Part print with two shaded views. Sizes in mm from the minimum x, y, z corner. Round coordinates to 2 decimals unless told otherwise and drop trailing zeros. Loops run counter-clockwise (first coordinate to the right, second up) from the corner with the lowest first, then second, coordinate; pieces in that order, holes last.
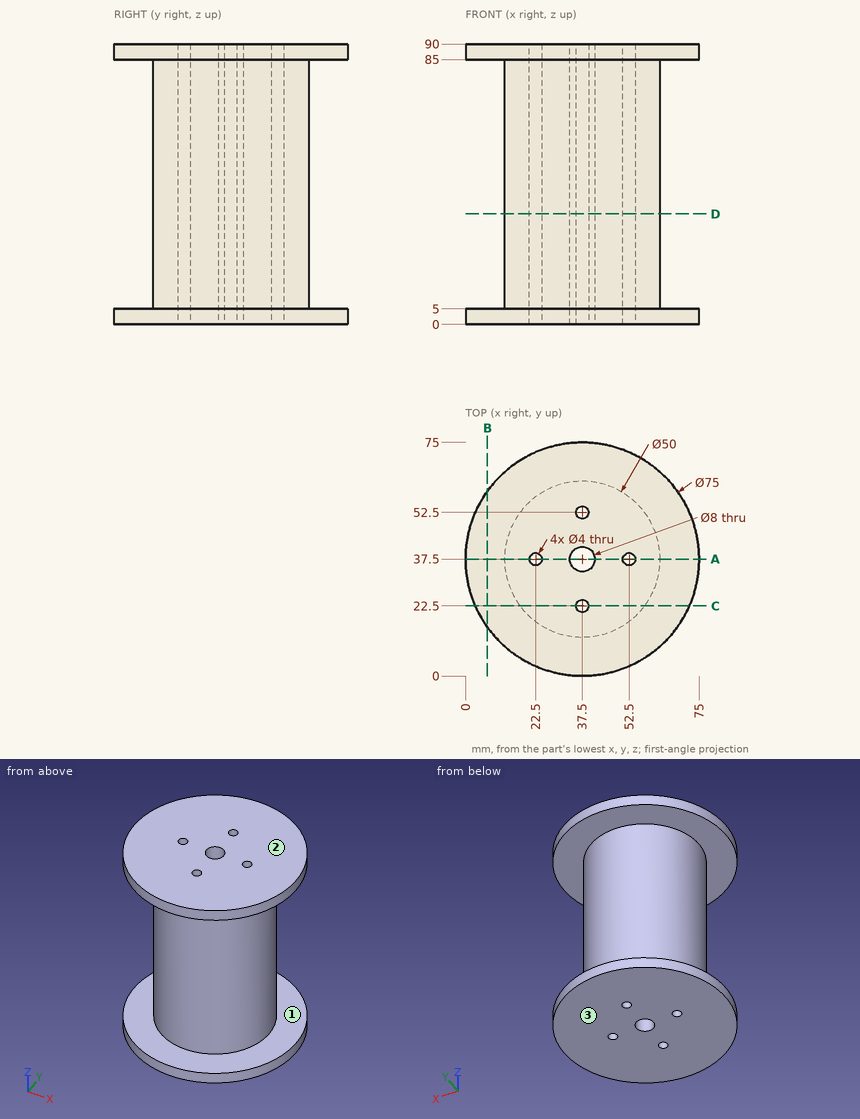
Item 1: Cut at B-B (x = 7). List the corners of the cut face in (y, z), plus the area to 3 significant figures.
Verdict:
outline: (15.68, 0) - (59.32, 0) - (59.32, 5) - (15.68, 5) - close; (15.68, 85) - (59.32, 85) - (59.32, 90) - (15.68, 90) - close
area: 436 mm2
Item 2: Flat gauge pins, fed straight in: P1, Ø13, axis at x = 37.5, y = 37.5, coming from the -Z side; P2, Ø8, axis at x = 11.5, z = 66.5, coming from the +Y side; P3, Ø6, axis at y = 23.5, z = 15, coming from the +X side; P4, Ø2, axis at x = 45, z = 37.5, coming from the +Y side. Where does each tip first touch, or does it go through?
Verdict:
P1: stops at z = 0
P2: stops at y = 49.37
P3: stops at x = 59.95
P4: stops at y = 61.64
Item 3: Cut at C-C (y = 22.5). List the corners of the cut face in (x, z).
Verdict:
outline: (3.13, 0) - (35.5, 0) - (35.5, 90) - (3.13, 90) - (3.13, 85) - (17.5, 85) - (17.5, 5) - (3.13, 5) - close; (39.5, 0) - (71.87, 0) - (71.87, 5) - (57.5, 5) - (57.5, 85) - (71.87, 85) - (71.87, 90) - (39.5, 90) - close
Item 4: Cut at D-D (z = 35.5). List the corners of the cut face in (x, y), plus the area to 3 significant figures.
Verdict:
outline: circle Ø50 at (37.5, 37.5); hole circle Ø4 at (22.5, 37.5); hole circle Ø8 at (37.5, 37.5); hole circle Ø4 at (37.5, 22.5); hole circle Ø4 at (37.5, 52.5); hole circle Ø4 at (52.5, 37.5)
area: 1,860 mm2
Item 5: Cut at A-A (y = 37.5). List the corners of the cut face in (x, z), plus the area to 3 significant figures.
Verdict:
outline: (0, 0) - (20.5, 0) - (20.5, 90) - (0, 90) - (0, 85) - (12.5, 85) - (12.5, 5) - (0, 5) - close; (24.5, 0) - (33.5, 0) - (33.5, 90) - (24.5, 90) - close; (41.5, 0) - (50.5, 0) - (50.5, 90) - (41.5, 90) - close; (54.5, 0) - (75, 0) - (75, 5) - (62.5, 5) - (62.5, 85) - (75, 85) - (75, 90) - (54.5, 90) - close
area: 3,310 mm2
Item 6: Mould opens along Z. For the marked faces 1, 2 and 3 say: released by +Z, released by -Z, zero draft, split by the parting line, or undercut.
Verdict:
face 1: undercut
face 2: released by +Z
face 3: released by -Z
Item 7: Wall check: L1, parallel to Y at x = 37.5, z = 60; L2, parallel to Y at x = 37, z = 21 (1 decimal). Give the ranges that are in metal, low to high.
Verdict:
L1: y = 12.5 to 20.5, 24.5 to 33.5, 41.5 to 50.5, 54.5 to 62.5
L2: y = 12.5 to 20.6, 24.4 to 33.5, 41.5 to 50.6, 54.4 to 62.5
